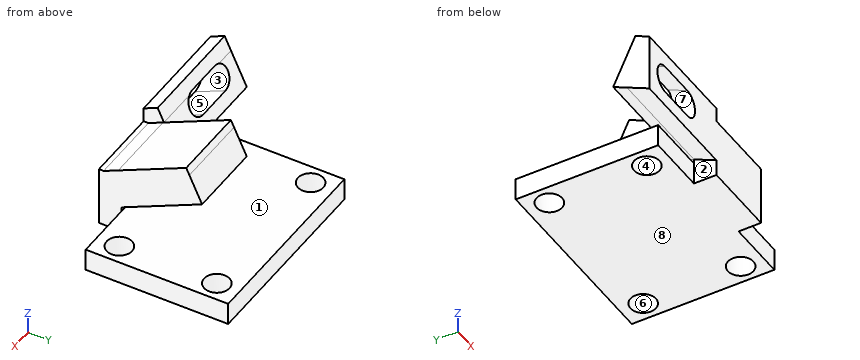
Autodesk Inventor part; units mm, degrees
ref_plane "YZ Plane" through (0, 0, 0) normal (1, 0, 0) x (0, 1, 0)
ref_plane "XZ Plane" through (0, 0, 0) normal (0, 1, 0) x (-1, 0, 0)
ref_plane "XY Plane" through (0, 0, 0) normal (0, 0, 1) x (1, 0, 0)
sketch "Sketch2" plane through (0, 0, 0) normal (0, 0, 1) x (1, 0, 0)
  line L0 (-13, -9.5) -> (13, -9.5)
  line L1 (13, -9.5) -> (13, 9.5)
  line L2 (13, 9.5) -> (-13, 9.5)
  line L3 (-13, 9.5) -> (-13, -9.5)
  line L4 (-13, -9.5) -> (13, 9.5) construction
  line L5 (13, -9.5) -> (-13, 9.5) construction
  point P0 (0, 0)
  dimension "d2" = 26
  dimension "d3" = 19
extrude "Extrusion1" add sketch "Sketch2" along normal blind 3
sketch "Sketch1" plane through (0, 0, 0) normal (0, 0, 1) x (1, 0, 0)
  line L0 (-10.5, -6.5) -> (10.5, -6.5) construction
  line L1 (10.5, -6.5) -> (10.5, 6.5) construction
  line L2 (10.5, 6.5) -> (-10.5, 6.5) construction
  line L3 (-10.5, 6.5) -> (-10.5, -6.5) construction
  line L4 (-10.5, -6.5) -> (10.5, 6.5) construction
  line L5 (10.5, -6.5) -> (-10.5, 6.5) construction
  point P0 (0, 0)
  dimension "d0" = 21
  dimension "d1" = 13
hole "Hole1" at (10.5, 6.5, 0) at (-10.5, 6.5, 0) at (10.5, -6.5, 0) at (-10.5, -6.5, 0) direction (0, 0, 1) diameter 3.4 end through all
sketch "Sketch3" plane through (0, 0, 0) normal (1, 0, 0) x (0, 1, 0)
  line L0 (-9.5, 0) -> (9.5, 0)
  line L1 (9.5, 0) -> (9.5, 3)
  line L2 (-9.5, 3) -> (9.5, 3)
  line L3 (-9.5, 0) -> (-9.5, 3)
  line L4 (-9.5, 0) -> (9.5, 0)
  line L5 (-9.5, 0) -> (-9.5, 8)
  line L6 (-9.5, 8) -> (-12.5, 8)
  line L7 (-12.5, 8) -> (-12.5, 0)
  line L8 (-12.5, 0) -> (-9.5, 0)
  line L9 (-9.5, 8) -> (-0.4369, 12.2262)
  line L10 (-0.4369, 12.2262) -> (1.2536, 8.601)
  line L11 (1.2536, 8.601) -> (-7.8095, 4.3748)
  line L12 (-7.8095, 4.3748) -> (-9.5, 8)
  line L13 (-9.5, 8) -> (0.5, 8) construction
  line L14 (-7.8095, 4.3748) -> (-9.5, 3.5865)
  line L15 (-0.4369, 12.2262) -> (-9.5, 8)
  line L16 (-9.5, 8) -> (-9.9226, 8.9063)
  line L17 (-9.9226, 8.9063) -> (-0.8595, 13.1325)
  line L18 (-0.8595, 13.1325) -> (-0.4369, 12.2262)
  line L19 (-9.9226, 8.9063) -> (-11.8662, 8)
  point P0 (0, 0)
  point P1 (-11, 8)
  dimension "d13" = 3
  dimension "d14" = 8
  dimension "d15" = 25
  dimension "d16" = 4
  dimension "d17" = 10
  dimension "d20" = 1
  dimension "d21" = 2.1445
extrude "Extrusion2" add sketch "Sketch3" along normal mid plane 10 contours L8 L7 L6 L5 L3 | L5 L12 L14 | L16 L17 L18 L9 | L9 L10 L11 L12 | L6 L19 L16
sketch "Sketch4" plane through (-5, 0, 0) normal (-1, 0, 0) x (0, 0, 1)
  line L0 (8.601, 1.2536) -> (3.5865, -9.5)
  line L1 (13.1325, -0.8595) -> (8, -11.8662)
  line L2 (4.4408, -7.668) -> (2.1876, -12.5)
  line L3 (0, -12.5) -> (8, -12.5)
  line L4 (9.5697, -8.5) -> (7.7045, -12.5)
  line L5 (7.7045, -12.5) -> (2.1876, -12.5)
  line L6 (4.4408, -7.668) -> (8.9723, -9.7811)
  line L7 (13.1325, -0.8595) -> (8.601, 1.2536)
  line L8 (8.9723, -9.7811) -> (10.7849, -10.6263)
  line L9 (10.7849, -10.6263) -> (9.9112, -12.5)
  line L10 (9.9112, -12.5) -> (7.7045, -12.5)
  line L11 (8, -11.8662) -> (8, -12.5)
  point P0 (0, 0)
  point P1 (8, -11.8662)
  point P2 (8, -11.8662)
  dimension "d25" = 3
  dimension "d33" = 2
extrude "Extrusion3" add sketch "Sketch4" along normal blind 15 contours L6 L1 L4 L3 L2 L0 | L8 L9 L10 L11 L1 | L11 L3 L4
sketch "Sketch6" plane through (-20, -7.668, 4.4408) normal (0, 0.9063, 0.4226) x (1, 0, 0)
  line L0 (3.5, -3.5) -> (8.5, -3.5) construction
  line L1 (3.5, -5.2) -> (8.5, -5.2)
  line L2 (8.5, -1.8) -> (3.5, -1.8)
  arc A0 (3.5, -1.8) -> (3.5, -5.2) centre (3.5, -3.5) ccw
  arc A1 (8.5, -5.2) -> (8.5, -1.8) centre (8.5, -3.5) ccw
  line L3 (0, -7) -> (0, 0)
  point P0 (20, 7.2653)
  point P1 (6, -3.5)
  point P2 (0, -3.5)
  dimension "d34" = 5
  dimension "d35" = 3.4
  dimension "d36" = 6
extrude "Extrusion5" cut sketch "Sketch6" against normal through all
properties part number "cam mount prototype"
Work out the finished part from the listing and answer in its coordinate system (mm). Face numbers are marked on the shaded views. A direction names the side the tool comes from. Give positions to 0.01 mm unless a question says otherwise; leave off trailing zeros. Order: outer loops, then holes, each group sorted by start corner. A loop starts at its lowest first (then second) coordinate and runs counter-clockwise, first axis right, second up. Notation, with made-up numbers: (52.25, -3.5) -> (68.25, -3.5) arc R24 cw to (68.25, 8.5) -> close; hole circle Ø7 at (36.5, 66.5). An arc over 180 degrees is marked (long way). Answer as a JSON object with one key per item and string values. Group by question number.
1. Section A-A on x = 10.5 is taken. Determine the outline of the cut face in (y, z).
2. Flat-ended cylindrical pins translate along their axes: pin 1 Ø3 at (y, z) = (-10.5, 9.5) entering from +X; pin 2 Ø5 at (x, y) = (-14.5, 3.5) entering from -Z; pin 3 Ø3.5 at (y, z) = (1.5, 1) entering from -X; pin 4 Ø3.5 at (x, z) = (7.5, 2) entering from -Y. Find the tip coordinate at first contact, or state that the pin passes through.
3. The mould has two halves that part along Z. Classify the marked faces 5, 6, 7 and 8: released by +Z, released by -Z, zero draft, split by the parting line, or undercut.
4. Section D-D on z = 10.25 is taken. Determine the outline of the cut face in (x, y), plus the area to 3 significant figures.
5. A tool of negligible diameter and unlimited length cuts with its end or side. For the marked faces 1, 2, 3 and 4, from which of +Z, -Z, +X, -X, +Y, -Y can it reach the whole face along a straight path? Write none if from no direction.
6. Section B-B on y = 6.5 is taken. Determine the outline of the cut face in (x, z).
7. Consider line 1 along Y through (x, z) = (10.5, 1.4); line 2 along X through (y, z) = (-6.5, 1.95); line 3 along X through (y, z) = (-1, 7.75). Determine where each line is inside the solid, lowest interval first. Write a range as [from, to].
8. Section C-C on x = -3.5 is taken. Determine the outline of the cut face in (y, z).
Result sheet:
{
 "1": {"outline": "(-9.5, 0) -> (-8.2, 0) -> (-8.2, 3) -> (-9.5, 3) -> close; (-4.8, 0) -> (4.8, 0) -> (4.8, 3) -> (-4.8, 3) -> close; (8.2, 0) -> (9.5, 0) -> (9.5, 3) -> (8.2, 3) -> close"},
 "2": {"pin 1": "stops at x = 5", "pin 2": "stops at z = 0", "pin 3": "stops at x = -13", "pin 4": "stops at y = -9.5"},
 "3": {"face 5": "undercut", "face 6": "zero draft", "face 7": "undercut", "face 8": "released by -Z"},
 "4": {"outline": "(-20, -11.77) -> (-5, -11.77) -> (-5, -10.38) -> (-20, -10.38) -> close; (-5, -7.04) -> (5, -7.04) -> (5, 0.48) -> (-5, 0.48) -> close", "area": "96.2 mm^2"},
 "5": {"face 1": "+X, -X, +Y", "face 2": "-Z, -X", "face 3": "none", "face 4": "-Z"},
 "6": {"outline": "(-13, 0) -> (-12.2, 0) -> (-12.2, 3) -> (-13, 3) -> close; (-8.8, 0) -> (8.8, 0) -> (8.8, 3) -> (-8.8, 3) -> close; (12.2, 0) -> (13, 0) -> (13, 3) -> (12.2, 3) -> close"},
 "7": {"line 1": "y = [-9.5, -8.2], [-4.8, 4.8], [8.2, 9.5]", "line 2": "x = [-13, -12.2], [-8.8, 8.8], [12.2, 13]", "line 3": "x = [-5, 5]"},
 "8": {"outline": "(-12.5, 0) -> (9.5, 0) -> (9.5, 3) -> (-9.5, 3) -> (-9.5, 3.59) -> (-7.81, 4.37) -> (1.25, 8.6) -> (-0.44, 12.23) -> (-0.86, 13.13) -> (-9.92, 8.91) -> (-11.87, 8) -> (-12.5, 8) -> close"}
}
